Source: CAD feature listing. Evaluate the final solid. Frame: model axes, mm. Round coordinates to 2 decimals unless told otherwise and drop trailing zeros. Order: outer loops, then holes, each group sorted by start corner. A loop starts at its lowest first (then second) coordinate and runs counter-clockwise, first axis right, second up.
```python
from build123d import *

# Parameters (mm, degrees)
SKETCH1_R           = 6.4
BOSS_EXTRUDE1_DEPTH = 2.1
SKETCH2_W           = 40.5
SKETCH2_H           = 19.8
BOSS_EXTRUDE2_DEPTH = 37.5


with BuildPart() as part:
    # Sketch1 → Boss-Extrude1 (new body)
    with BuildSketch(Plane(origin=(0, 0, 0), x_dir=(1, 0, 0), z_dir=(0, 1, 0))):
        with Locations(Location((0, 0, 0), (0, 0, 270))):
            Circle(SKETCH1_R)
    extrude(amount=BOSS_EXTRUDE1_DEPTH)

    # Sketch2 → Boss-Extrude2 (add)
    with BuildSketch(Plane.XZ):
        with Locations((10.35, 0)):
            Rectangle(SKETCH2_W, SKETCH2_H)
    extrude(amount=BOSS_EXTRUDE2_DEPTH)


solid = part.part
```
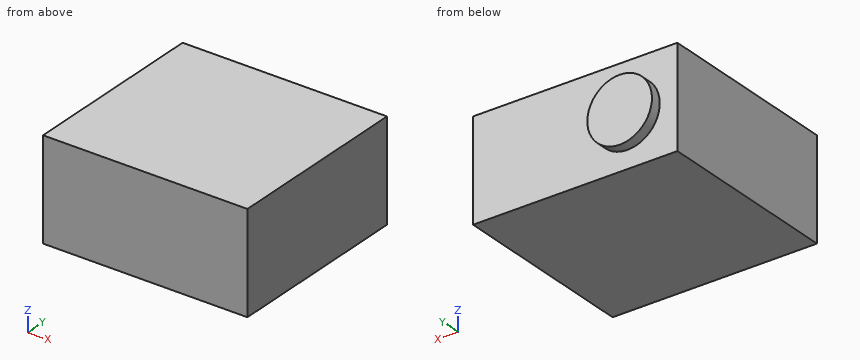
1. Line query: line 1 along Y through (x, z) = (7, -1.5). Output: solid intervals per line, ascending.
2. Section C-C on z = 7. Return loops of the section in (x, y).
3. First-contact query: pin 1 (3 mm diameter, centred on x = 10.5, z = -4, fed in from +Y). Flat tip, straight axial feed; report the tip coordinate or a pass-through.
4. Section D-D on x = 21. Return loops of the section in (y, z), plus the area to 4 significant figures.
5. Section B-B on z = 0. Return loops of the section in (x, y).
6. Section A-A on x = 3. Return loops of the section in (y, z).
Result:
1. line 1: y = -37.5 to 0
2. outline: (-9.9, -37.5) - (30.6, -37.5) - (30.6, 0) - (-9.9, 0) - close
3. pin 1: stops at y = 0
4. outline: (-37.5, -9.9) - (0, -9.9) - (0, 9.9) - (-37.5, 9.9) - close
4. area: 742.5 mm2
5. outline: (-9.9, -37.5) - (30.6, -37.5) - (30.6, 0) - (6.4, 0) - (6.4, 2.1) - (-6.4, 2.1) - (-6.4, 0) - (-9.9, 0) - close
6. outline: (-37.5, -9.9) - (0, -9.9) - (0, -5.65) - (2.1, -5.65) - (2.1, 5.65) - (0, 5.65) - (0, 9.9) - (-37.5, 9.9) - close
